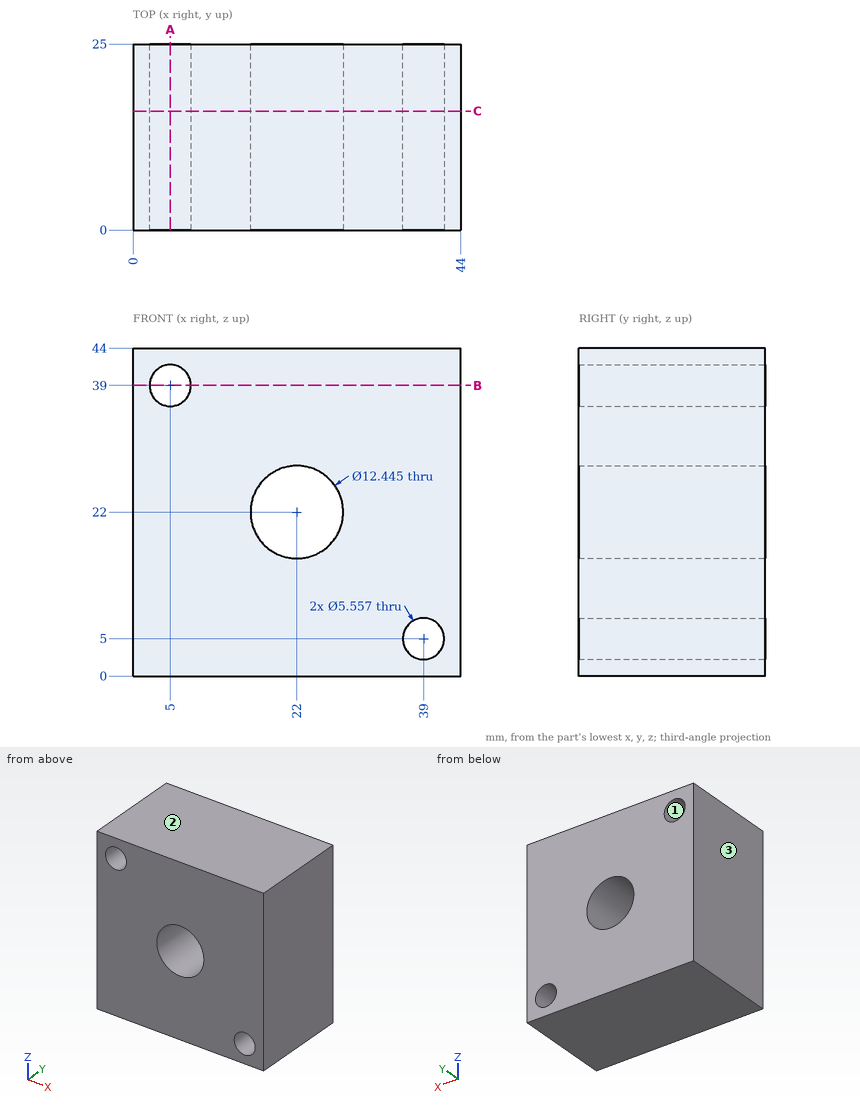
The drawing under review shows one solid part. Ordinate dimensions are in mm from its lowest x, y, z. Give positions to 0.01 mm unless a question says otherwise; leave off trailing zeros. Write each loop counter-clockwise with the first axis right and the second up, starting at its lowest first coordinate (ties: lowest second). Pieces come first, ordered by that corner, then holes. Notation, with made-up numbers: M 10,-32 L 23,-32 A16 cw 23,-19 Z; hole C -30.75,33 d7. An arc over 180 degrees is marked long. Write each question's results on one line, items separated by ' | '. Start each with the question number.
1. Mouldability with a two-part tool opening along Z and no side actions: class the marked faces 1, 2 and 3 as released by +Z, released by -Z, zero draft, split by the parting line, or undercut.
2. We need section C-C (y = 16). Write out the cut boundary in (x, z) (1 decimal).
3. For probe 1 along Z at (x, y) = (5, 7.5); probe 2 along Z at (x, y) = (39, 19.25); probe 3 along X at (y, z) = (4.5, 20), list the stretches that pass through material, from the lowest coordinate up. Write a range as [from, to].
4. We need section B-B (z = 39). Write out the cut boundary in (x, y), and give its area (3 significant figures).
5. Insertion check: pin 1 Ø10 at (x, z) = (22, 22) entering from -Y. The pin has a flat end and moves straight along its axis. Give the tip position at first contact, or say it passes through.
6. We need section A-A (x = 5). Write out the cut boundary in (y, z), and give its area (3 significant figures).
Results found:
1) face 1: undercut | face 2: released by +Z | face 3: zero draft
2) outline: M 0,0 L 44,0 L 44,44 L 0,44 Z; hole C 5,39 d5.6; hole C 22,22 d12.4; hole C 39,5 d5.6
3) probe 1: z = [0, 36.22], [41.78, 44] | probe 2: z = [0, 2.22], [7.78, 44] | probe 3: x = [0, 16.11], [27.89, 44]
4) outline: M 0,0 L 2.22,0 L 2.22,25 L 0,25 Z; M 7.78,0 L 44,0 L 44,25 L 7.78,25 Z | area: 961 mm^2
5) pin 1: passes through
6) outline: M 0,0 L 25,0 L 25,36.22 L 0,36.22 Z; M 0,41.78 L 25,41.78 L 25,44 L 0,44 Z | area: 961 mm^2
